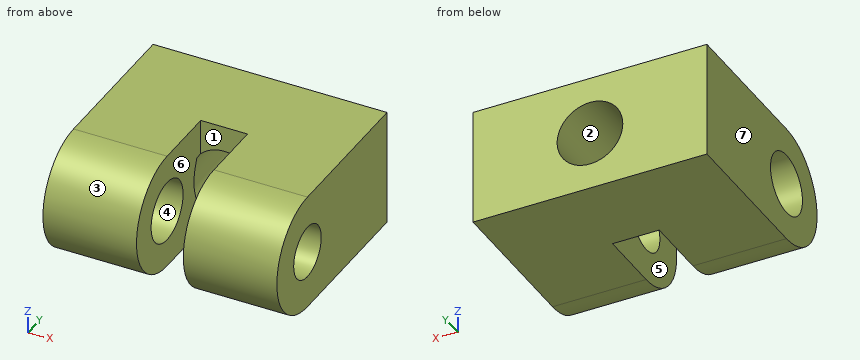
from build123d import *

# Parameters (mm, degrees)
SKETCH1_W                       = 20
SKETCH1_H                       = 10
BOSS_EXTRUDE1_DEPTH             = 18
CUT_EXTRUDE1_DEPTH              = 22.1896201
CUT_EXTRUDE1_DEPTH_BACK         = 22.1896201
SKETCH2_W                       = 4
SKETCH2_H                       = 10.5
F_16_0_177_DIAMETER_HOLE1_D     = 4.4958
F_16_0_177_DIAMETER_HOLE1_DEPTH = 8
SKETCH6_W                       = 2.60985
SKETCH6_H                       = 8
F_2_0_221_DIAMETER_HOLE1_D      = 5.6134
F_2_0_221_DIAMETER_HOLE1_DEPTH  = 8.128
F_2_0_221_DIAMETER_HOLE1_TIP    = 1.686435499
FILLET2_RADIUS                  = 5
FILLET2_LENGTH                  = 8
FILLET3_RADIUS                  = 5
FILLET3_LENGTH                  = 8


with BuildPart() as part:
    # Sketch1 → Boss-Extrude1 (new body)
    with BuildSketch(Plane(origin=(0, 0, 0), x_dir=(1, 0, 0), z_dir=(0, 1, 0))):
        Rectangle(SKETCH1_W, SKETCH1_H)
    extrude(amount=BOSS_EXTRUDE1_DEPTH)

    # Sketch2 → Cut-Extrude1 (cut, two sides: drawn at the far end of the back side and taken through both)
    with BuildSketch(Plane.XY.offset(-CUT_EXTRUDE1_DEPTH_BACK)):
        with Locations((0, 5.25)):
            Rectangle(SKETCH2_W, SKETCH2_H)
    extrude(amount=CUT_EXTRUDE1_DEPTH + CUT_EXTRUDE1_DEPTH_BACK, mode=Mode.SUBTRACT)

    # #16 (0.177) Diameter Hole1
    with Locations(Plane(origin=(10, 0, 0), x_dir=(0, 0, -1), z_dir=(1, 0, 0))):
        with Locations((0, 5)):
            Hole(F_16_0_177_DIAMETER_HOLE1_D / 2, depth=F_16_0_177_DIAMETER_HOLE1_DEPTH)

    # Sketch6 → #5 (0.2055) Diameter Hole1 (revolve, cut)
    with BuildSketch(Plane(origin=(-2, 5, 0), x_dir=(0, 0, -1), z_dir=(0, 1, 0))):
        with Locations((1.304925, 4)):
            Rectangle(SKETCH6_W, SKETCH6_H)
    revolve(axis=Axis((4.35, 5, 0), (-1, 0, 0)), mode=Mode.SUBTRACT)

    # #2 (0.221) Diameter Hole1
    with Locations(Plane(origin=(0, 18, 0), x_dir=(1, 0, 0), z_dir=(0, 1, 0))):
        with Locations((0, 0)):
            Hole(F_2_0_221_DIAMETER_HOLE1_D / 2, depth=F_2_0_221_DIAMETER_HOLE1_DEPTH)
            with Locations((0, 0, -(F_2_0_221_DIAMETER_HOLE1_DEPTH + F_2_0_221_DIAMETER_HOLE1_TIP / 2))):  # 118° drill point
                Cone(0, F_2_0_221_DIAMETER_HOLE1_D / 2, F_2_0_221_DIAMETER_HOLE1_TIP, mode=Mode.SUBTRACT)

    # Fillet2: full round fillet: the end face becomes a half cylinder, R = half its width
    fillet2_face = Plane((-6, 0, 0), x_dir=(1, 0, 0), z_dir=(0, -1, 0))  # on the end face: x along it, z out of the body
    fillet2_slab = fillet2_face.offset(-FILLET2_RADIUS / 2) * Box(FILLET2_LENGTH, 2 * FILLET2_RADIUS, FILLET2_RADIUS, mode=Mode.PRIVATE)  # the body's end, R deep
    fillet2_round = Plane((-6, 5, 0), x_dir=(0, -1, 0), z_dir=(1, 0, 0)) * Cylinder(FILLET2_RADIUS, FILLET2_LENGTH, mode=Mode.PRIVATE)  # its axis R under the face
    add(fillet2_slab - fillet2_round, mode=Mode.SUBTRACT)

    # Fillet3: full round fillet: the end face becomes a half cylinder, R = half its width
    fillet3_face = Plane((6, 0, 0), x_dir=(-1, 0, 0), z_dir=(0, -1, 0))  # on the end face: x along it, z out of the body
    fillet3_slab = fillet3_face.offset(-FILLET3_RADIUS / 2) * Box(FILLET3_LENGTH, 2 * FILLET3_RADIUS, FILLET3_RADIUS, mode=Mode.PRIVATE)  # the body's end, R deep
    fillet3_round = Plane((6, 5, 0), x_dir=(0, -1, 0), z_dir=(-1, 0, 0)) * Cylinder(FILLET3_RADIUS, FILLET3_LENGTH, mode=Mode.PRIVATE)  # its axis R under the face
    add(fillet3_slab - fillet3_round, mode=Mode.SUBTRACT)


solid = part.part
Design review of the part built by this model. Coordinates are the model's own, in mm. Face numbers are marked on the shaded views. A direction names the side the tool comes from. Give positions to 0.01 mm unless a question says otherwise; leave off trailing zeros. Loops run counter-clockwise (first coordinate to the right, second up) from the corner with the lowest first, then second, coordinate; pieces in that order, holes last. Notation, with made-up numbers: M 49.25,15 L 89.25,15 A22 ccw 89.25,23 Z; hole C 36.25,-31.75 d5. An arc over 180 degrees is marked long. Write item = value, one per line.
Q1. We need section B-B (y = 8). Give the boundary of the cut face in (x, z).
Output values:
outline = M -10,-5 L -2,-5 L -2,5 L -10,5 Z; M 2,-5 L 10,-5 L 10,5 L 2,5 Z
Q2. Draft analysis for pull direction X (two halves, no side actions). For the marked faces 4, 5, 6 and 7, state which applies: +X half, -X half, draft (parallel to the pull), parting line (faces both ways), or undercut.
Output values:
face_4 = draft
face_5 = undercut
face_6 = undercut
face_7 = -X half
Q3. We need section C-C (z = 4). Give the boundary of the cut face in (x, y), plus the area to 3 significant figures.
Output values:
outline = M -10,2 L -2,2 L -2,10.5 L 2,10.5 L 2,2 L 10,2 L 10,18 L -10,18 Z
area = 286 mm^2
Q4. For the marked faces 1, 2 and 3, list the 3-axis set-ups (+Z, -Z, +X, -X, +Y, -Y) from which the entire face can be reached by the end or side of a thin tool; tool diameter is ignored.
Output values:
face_1 = +Z, -Z, -Y
face_2 = +Y
face_3 = +X, -X, -Y
Q5. Insertion check: pin 1 (2 mm diameter, centred on x = 3, z = 1.5, fed in from -Y); pin 2 (1.5 mm diameter, centred on x = -0.5, z = -3, fed in from -Y). Each pin has a flat end and moves straight along its axis. Give the tip position at first contact, or say it passes through.
Output values:
pin_1 = 0.03
pin_2 = 10.5
Q6. We need section D-D (x = -5.5). Give the boundary of the cut face in (y, z).
Output values:
outline = M 5,-5 L 18,-5 L 18,5 L 5,5 A5 ccw Z; hole C 5,0 d5.22
Q7. To check wall thickness, follow line 1 (Z direction, x = -7.5, y = 5); line 2 (Y direction, x = -6.75, z = 0); line 3 (X direction, y = 3, z = 2.75). State the ranges of each line that lie inside material, in increasing order. Write a range as [from, to].
Output values:
line_1 = [-5, -2.61], [2.61, 5]
line_2 = [0, 2.39], [7.61, 18]
line_3 = [-10, -2], [2, 10]
Q8. We need section A-A (x = 0). Give the boundary of the cut face in (y, z).
Output values:
outline = M 10.5,-5 L 18,-5 L 18,-2.81 L 10.5,-2.81 Z; M 10.5,2.81 L 18,2.81 L 18,5 L 10.5,5 Z
